```python
from build123d import *

# Parameters (mm, degrees)
F1_DEPTH = 25.4
F0_R     = 15.875
F2_DEPTH = 53.975
F0_W     = 31.75
F0_H     = 88.9
F3_DEPTH = 73.025
F0_H_2   = 31.75
F4_DEPTH = 92.075


# Not quite as in the source:
# - a feature names something its author has since deleted; it is built from what else it names


with BuildPart() as f1:
    # F0 (on Top) → F1 (new body)
    with BuildSketch(Plane.XY):
        Polygon((-75.5807677343, 77.5184368145), (-132.7307677343, 77.5184368145), (-132.7307677343, 26.7184368145), (-91.4557677343, 26.7184368145), (-91.4557677343, -24.0815631855), (-132.7307677343, -24.0815631855), (-132.7307677343, -74.8815631855), (-75.5807677344, -74.8815631855), (-75.5807677343, -43.1315631855), (-75.5807677343, 45.7684368145), align=None)
    extrude(amount=F1_DEPTH)



with BuildPart() as f1b:
    # F0 (on Top) → F1, piece 2 (new body)
    with BuildSketch(Plane.XY):
        Polygon((121.2692322657, 77.5184368145), (64.1192322657, 77.5184368145), (64.1192322657, 45.7684368145), (64.1192322657, -43.1315631855), (64.1192322657, -74.8815631855), (121.2692322657, -74.8815631855), (121.2692322657, -24.0815631855), (79.9942322657, -24.0815631855), (79.9942322657, 26.7184368145), (121.2692322657, 26.7184368145), align=None)
    extrude(amount=F1_DEPTH)


with BuildPart() as f2:
    # F0 (on Top) → F2 (new body)
    with BuildSketch(Plane.XY):
        Polygon((32.3692322657, 77.5184368145), (-43.8307677343, 77.5184368145), (-43.8307677343, 45.7684368145), (-43.8307677343, -43.1315631855), (-43.8307677343, -74.8815631855), (32.3692322657, -74.8815631855), (32.3692322657, -43.1315631855), (32.3692322657, 45.7684368145), align=None)
        with Locations((-5.7307677343, 1.3184368145)):
            Circle(F0_R, mode=Mode.SUBTRACT)
    extrude(amount=F2_DEPTH)


with BuildPart() as f1_1:
    add(f1.part)

    add(f1b.part)  # F3 merges F1b

    add(f2.part)  # F3 merges F2
    # F0 (on Top) → F3 (join)
    with BuildSketch(Plane.XY):
        with Locations((-59.7057677343, 1.3184368145)):
            Rectangle(F0_W, F0_H)
        with Locations((48.2442322657, 1.3184368145)):
            Rectangle(F0_W, F0_H)
    extrude(amount=F3_DEPTH)

    # F0 (on Top) → F4 (join)
    with BuildSketch(Plane.XY):
        with Locations((-59.7057677343, 61.6434368145)):
            Rectangle(F0_W, F0_H_2)
        with Locations((48.2442322657, 61.6434368145)):
            Rectangle(F0_W, F0_H_2)
        with Locations((-59.7057677343, -59.0065631855)):
            Rectangle(F0_W, F0_H_2)
        with Locations((48.2442322657, -59.0065631855)):
            Rectangle(F0_W, F0_H_2)
    extrude(amount=F4_DEPTH)


solid = f1_1.part
```
CAD build for the part. Positions are in the model's coordinates, mm. A direction names the side the tool comes from. Give positions to 0.01 mm unless a question says otherwise; leave off trailing zeros. Order: outer loops, then holes, each group sorted by start corner. A loop starts at its lowest first (then second) coordinate and runs counter-clockwise, first axis right, second up.
(1) Flat gauge pins, fed straight in: pin 1 (11.5 mm diameter, centred on y = 31.5, z = 76.5, fed in from +X); pin 2 (8 mm diameter, centred on x = -32.5, y = 58.5, fed in from +Z) (3 decimals); pin 3 (19 mm diameter, centred on x = -5.73, y = 1.32, fed in from -Z); pin 4 (17 mm diameter, centred on x = 85, y = 33, fed in from +Z). Where does each tip first touch, or does it go through?
(2) Saw through at D-D, the plane x = 49.5. Give the cut face in (y, z) (3 decimals).
(3) Mould opens along X. For faces 4 (the flat face through (121.269, -50, 13)), 5 (the flat face through (-60, 2, 73.025)), 6 (the flat face through (-132.731, -49, 13)), 7 (the flat face through (32.369, 0, 69)) say: released by +X, released by -X, zero draft, split by the parting line, or undercut.
(4) Saw through at A-A, the plane z = 57. Give the cut face in (x, y), then the cut area to 3 significant figures.
(5) Saw through at C-C, the plane y = -37. Give the cut face in (x, z) (3 decimals).
(6) Tool access for faces 1 (the flat face through (-43.831, 0, 69)), 2 (the flat face through (-60, 45.768, 82)), 3 (the flat face through (-112, -24.082, 13)): list every direction of +Z, -Z, +X, -X, +Y, -Y with a clear straight run to the whole face (end or side of a thin tool).
(7) Saw through at B-B, the plane x = 100. Give the cut face in (y, z).
(8) Drill centre lines: L1, parallel to X at y = -64, z = 66; L2, parallel to Y at x = 44.5, z = 85; L3, parallel to Y at x = -98.5, z = 17.5. Where is each one in solid material? Low to high.
Results found:
1. pin 1: stops at x = 64.12
1. pin 2: stops at z = 53.975
1. pin 3: passes through
1. pin 4: stops at z = 25.4
2. outline: (-74.882, 0) - (77.518, 0) - (77.518, 92.075) - (45.768, 92.075) - (45.768, 73.025) - (-43.132, 73.025) - (-43.132, 92.075) - (-74.882, 92.075) - close
3. face 4: released by +X
3. face 5: zero draft
3. face 6: released by -X
3. face 7: undercut
4. outline: (-75.58, -74.88) - (-43.83, -74.88) - (-43.83, 77.52) - (-75.58, 77.52) - close; (32.37, -74.88) - (64.12, -74.88) - (64.12, 77.52) - (32.37, 77.52) - close
4. area: 9,680 mm2
5. outline: (-132.731, 0) - (121.269, 0) - (121.269, 25.4) - (64.119, 25.4) - (64.119, 73.025) - (32.369, 73.025) - (32.369, 53.975) - (-43.831, 53.975) - (-43.831, 73.025) - (-75.581, 73.025) - (-75.581, 25.4) - (-132.731, 25.4) - close
6. face 1: +Z, +Y, -Y
6. face 2: +Z, +X, -X
6. face 3: +Z, -Z, -X
7. outline: (-74.88, 0) - (-24.08, 0) - (-24.08, 25.4) - (-74.88, 25.4) - close; (26.72, 0) - (77.52, 0) - (77.52, 25.4) - (26.72, 25.4) - close
8. L1: x = -75.58 to -43.83, 32.37 to 64.12
8. L2: y = -74.88 to -43.13, 45.77 to 77.52
8. L3: y = -74.88 to -24.08, 26.72 to 77.52
